Print and shaded views of the part. All mm, measured from the part's lowest x, y and z. A direction names the side the tool comes from. Give positions to 0.01 mm unless a question says otherwise; leave off trailing zeros. Loops run counter-clockwise (first coordinate to the right, second up) from the corner with the lowest first, then second, coordinate; pieces in that order, holes last. Notation, with made-up numbers: M 42.25,0 L 78.25,0 A18 cw 78.25,5 Z; hole C 36,85 d7. An arc over 180 degrees is marked long. Answer in a Markdown table with one row per item.
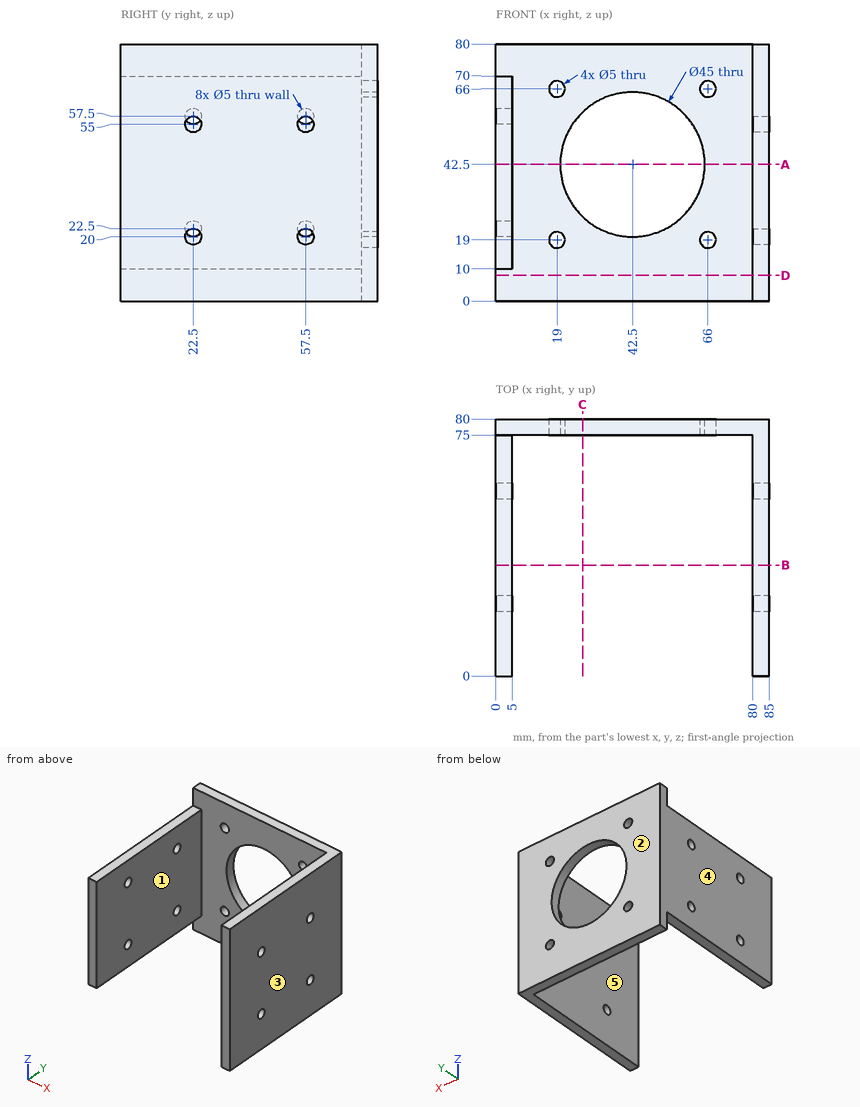
(1) Wall check: L1, parallel to Y at x = 1.75, z = 57.5; L2, parallel to Z at x = 19, y = 78.25; L3, parallel to X at y = 18, z = 37. Give the ranges that are in metal, low to high.
Established:
| item | result |
|---|---|
| L1 | y = 0 to 20, 25 to 55, 60 to 80 |
| L2 | z = 0 to 16.5, 21.5 to 63.5, 68.5 to 80 |
| L3 | x = 0 to 5, 80 to 85 |
(2) Saw through at B-B, the plane y = 34.5. Give the cut face in (x, z), and give its area (3 significant figures).
Established:
| item | result |
|---|---|
| outline | M 0,10 L 5,10 L 5,70 L 0,70 Z; M 80,0 L 85,0 L 85,80 L 80,80 Z |
| area | 700 mm2 |
(3) Flat gauge pins, fed straight in: P1, Ø6, axis at y = 22.5, z = 22.5, coming from the -X side; P2, Ø4, axis at x = 3.5, y = 22, coming from the -Z side; P3, Ø4.5, axis at x = 66, z = 19, coming from the +Y side; P4, Ø4, axis at y = 22.5, z = 55, coming from the +X side. Where does each tip first touch, or does it go through?
Established:
| item | result |
|---|---|
| P1 | stops at x = 0 |
| P2 | stops at z = 10 |
| P3 | passes through |
| P4 | stops at x = 5 |
(4) Saw through at A-A, the plane z = 42.5. Give the cut face in (x, y), and give its area (3 significant figures).
Established:
| item | result |
|---|---|
| outline | M 0,0 L 5,0 L 5,75 L 20,75 L 20,80 L 0,80 Z; M 65,75 L 80,75 L 80,0 L 85,0 L 85,80 L 65,80 Z |
| area | 950 mm2 |
(5) Mould opens along X. For the marked faces 3, 4 and 5 say: pulls with the +X half, pulls with the -X half, needs draft (parallel to the pull), parting line crosses it, or undercut.
Established:
| item | result |
|---|---|
| face 3 | pulls with the +X half |
| face 4 | pulls with the -X half |
| face 5 | undercut |
(6) Saw through at D-D, the plane z = 8. Give the cut face in (x, y).
Established:
| item | result |
|---|---|
| outline | M 0,75 L 80,75 L 80,0 L 85,0 L 85,80 L 0,80 Z |
(7) Saw through at C-C, the plane x = 27. Give the cut face in (y, z), and give its area (3 significant figures).
Established:
| item | result |
|---|---|
| outline | M 75,0 L 80,0 L 80,26.19 L 75,26.19 Z; M 75,58.81 L 80,58.81 L 80,80 L 75,80 Z |
| area | 237 mm2 |
(8) Which spindle directions (+Z, -Z, +X, -X, +Y, -Y) get a long thin tool onto all of the face, cutting with end or side? Do the marked faces 1 and 2. Say none if no direction does.
Established:
| item | result |
|---|---|
| face 1 | +Z, -Z, -Y |
| face 2 | +Z, -Z, +X, -X, +Y |
